Autodesk Inventor part; units mm, degrees
ref_plane "YZ Plane" through (0, 0, 0) normal (1, 0, 0) x (0, 1, 0)
ref_plane "XZ Plane" through (0, 0, 0) normal (0, 1, 0) x (-1, 0, 0)
ref_plane "XY Plane" through (0, 0, 0) normal (0, 0, 1) x (1, 0, 0)
sketch "Esquisse1" plane through (0, 0, 0) normal (0, 0, 1) x (1, 0, 0)
  line L0 (0, 25) -> (146, 25)
  line L1 (146, 25) -> (146, 22)
  line L2 (146, 22) -> (0, 22)
  line L3 (0, 22) -> (0, 25)
  line L4 (-10.0826, 0) -> (43.679, 0)
  line L5 (-41.2991, 0) -> (177.2165, 0)
  line L6 (0, -5) -> (0, 30)
  point P0 (0, 0)
  dimension "d0" = 3
  dimension "d1" = 50
  dimension "d2" = 146
revolve "Révolution1" add sketch "Esquisse1" angle 360 about axis through (-10.0826, 0, 0) along (1, 0, 0)
sketch "Esquisse5" plane through (146, 0, 0) normal (1, 0, 0) x (0, 0, -1)
  line L0 (-35, 0) -> (35, 0) construction
  circle A0 centre (0, 0) radius 22 construction
  circle A1 centre (0, 0) radius 25 construction
  line L1 (-25, -21.6089) -> (-25, 34.5668) construction
  line L2 (-22, -18.8661) -> (-22, 30.8732) construction
  line L3 (-7, -26.0436) -> (-7, 26.1117) construction
  arc A2 (0, 22) -> (0, 22) centre (0, 0) ccw
  arc A3 (-7, 20.8567) -> (-7, -20.8567) centre (0, 0) ccw
  arc A4 (0, 25) -> (0, 25) centre (0, 0) ccw
  arc A5 (0, 25) -> (0, 25) centre (0, 0) ccw
  arc A6 (-7, 24) -> (-7, -24) centre (0, 0) ccw
  line L4 (-7, -24) -> (-7, -20.8567)
  line L5 (-7, 20.8567) -> (-7, 24)
  dimension "d31" = 15
extrude "Extrusion5" cut sketch "Esquisse5" against normal blind 100 contours A2 L4 A4 L5 picked at (-22.7161, 2.7828)
properties part number "S1702_tubeexterne" material "Plastique PMMA"
Read the model definition and answer for the solid it produces. Units are mm, in the model's axes. A direction names the side the tool comes from. Give positions to 0.01 mm unless a question says otherwise; leave off trailing zeros. Write each loop counter-clockwise with the first axis right and the second up, starting at its lowest first coordinate (ties: lowest second). Pieces come first, ordered by that corner, then holes. Notation, with made-up numbers: M -15,-20 L 30,-20 A19 ccw 30,13 Z; hole C 3,-15.5 d6. An arc over 180 degrees is marked long. One line per item, written item: value. Start each with the question number.
(1) A tool of negligible diameter and unlimited length cuts with its end or side. For faces 1 (the flat face through (97, 22, 7)), 2 (the flat face through (0, 1.7, -22.1)), from which of +Z, -Z, +X, -X, +Y, -Y can it reach the whole face along a straight path? Write none if from no direction.
(2) Find the intervals of material crossed by line 1 (Y direction, x = 68, z = 0); line 2 (Y direction, x = 118, z = -17), in increasing order.
(3) Determine the mould class of faces 3 (the flat face through (97, -22, 7)), 4 (the flat face through (46, 2, 23)), 5 (the cylindrical face through (55.756, -2.864, -21.813)), 6 (the cylindrical face through (57.8, -5.42, -24.406)) for opening direction Z: pulls with the +Z half, pulls with the -Z half, needs draft (parallel to the pull), parting line crosses it, or undercut.
(4) Find section C-C (x = 136.5). Determine the outline of the cut face in (y, z).
(5) Find section A-A (y = 0). Determine the outline of the cut face in (x, z), plus the area to 3 significant figures.
(6) Flat-ended cylindrical pins translate along their axes: pin 1 Ø3.5 at (x, y) = (88, -22) entering from +Z; pin 2 Ø10 at (x, y) = (50, 12.5) entering from +Z; pin 3 Ø2 at (x, z) = (30, -9.5) entering from +Y. Find the tip coordinate at first contact, or state that the pin passes through.
(7) Find section B-B (z = 0). Determine the outline of the cut face in (x, y), plus the area to 3 significant figures.
Results below:
1. face 1: +Z, +X, +Y, -Y
1. face 2: +Z, -Z, -X, +Y, -Y
2. line 1: y = -25 to -22, 22 to 25
2. line 2: y = -18.33 to -13.96, 13.96 to 18.33
3. face 3: pulls with the +Z half
3. face 4: needs draft
3. face 5: undercut
3. face 6: parting line crosses it
4. outline: M -24,7 A25 ccw long 24,7 L 20.86,7 A22 cw long -20.86,7 Z
5. outline: M 0,-25 L 146,-25 L 146,-22 L 0,-22 Z; M 0,22 L 46,22 L 46,25 L 0,25 Z
5. area: 576 mm^2
6. pin 1: stops at z = 7
6. pin 2: stops at z = 23.12
6. pin 3: stops at y = 23.51
7. outline: M 0,-25 L 146,-25 L 146,-22 L 0,-22 Z; M 0,22 L 146,22 L 146,25 L 0,25 Z
7. area: 876 mm^2
